```python
from build123d import *

# Parameters (mm, degrees)
F0_W      = 558.8
F0_H      = 330.2
F1_DEPTH  = 19.05
F2_W      = 38.1
F2_H      = 419.1
F2_H_2    = 203.2
F2_H_3    = 330.2
F3_DEPTH  = 88.9
F4_W      = 88.9
F4_H      = 88.9
F5_DEPTH  = 914.4
F6_W      = 38.1
F6_H      = 431.8
F6_W_2    = 431.8
F6_H_2    = 38.1
F7_DEPTH  = 139.7
F8_W      = 431.8
F8_H      = 69.85
F9_DEPTH  = 78.74
F10_W     = 431.8
F10_H     = 69.85
F11_DEPTH = 66.04
F12_W     = 431.8
F12_H     = 69.85
F13_DEPTH = 53.34
F14_W     = 431.8
F14_H     = 69.85
F15_DEPTH = 76.2


with BuildPart() as f1:
    # F0 (on Top) → F1 (new body)
    with BuildSketch(Plane.XY):
        Polygon((-907.6019599199, 71.2758600712), (-298.0019599199, -538.3241399288), (311.5980400801, -538.3241399288), (921.1980400801, 71.2758600712), (921.1980400801, 680.8758600712), (311.5980400801, 1290.4758600712), (-298.0019599199, 1290.4758600712), (-907.6019599199, 680.8758600712), align=None)
        with Locations((6.7980400801, 274.4758600712)):
            Rectangle(F0_W, F0_H, mode=Mode.SUBTRACT)
    extrude(amount=F1_DEPTH)

    # F2 (on face) → F3 (join)
    with BuildSketch(Plane(origin=(0, 0, 0), x_dir=(1, 0, 0), z_dir=(0, 0, -1))):
        with Locations((-278.9519599199, -890.4258600712)):
            Rectangle(F2_W, F2_H)
        with Locations((292.5480400801, -890.4258600712)):
            Rectangle(F2_W, F2_H)
        Polygon((-717.1019599199, -642.7758600712), (-717.1019599199, -680.8758600712), (-298.0019599199, -680.8758600712), (-259.9019599199, -680.8758600712), (273.4980400801, -680.8758600712), (311.5980400801, -680.8758600712), (730.6980400801, -680.8758600712), (730.6980400801, -642.7758600712), (273.4980400801, -642.7758600712), (235.3980400801, -642.7758600712), (-221.8019599199, -642.7758600712), (-259.9019599199, -642.7758600712), align=None)
        with Locations((-240.8519599199, -541.1758600712)):
            Rectangle(F2_W, F2_H_2)
        Polygon((-298.0019599199, -71.2758600712), (-717.1019599199, -71.2758600712), (-717.1019599199, -109.3758600712), (-272.6019599199, -109.3758600712), (-259.9019599199, -109.3758600712), (-221.8019599199, -109.3758600712), (235.3980400801, -109.3758600712), (273.4980400801, -109.3758600712), (286.1980400801, -109.3758600712), (730.6980400801, -109.3758600712), (730.6980400801, -71.2758600712), (311.5980400801, -71.2758600712), (273.4980400801, -71.2758600712), (-259.9019599199, -71.2758600712), align=None)
        with Locations((-278.9519599199, 138.2741399288)):
            Rectangle(F2_W, F2_H)
        with Locations((292.5480400801, 138.2741399288)):
            Rectangle(F2_W, F2_H)
        with Locations((254.4480400801, -541.1758600712)):
            Rectangle(F2_W, F2_H_2)
        with Locations((-240.8519599199, -274.4758600712)):
            Rectangle(F2_W, F2_H_3)
        with Locations((254.4480400801, -274.4758600712)):
            Rectangle(F2_W, F2_H_3)
    extrude(amount=F3_DEPTH)

    # F4 (on face) → F5 (join)
    with BuildSketch(Plane(origin=(0, 0, 0), x_dir=(1, 0, 0), z_dir=(0, 0, -1))):
        with Locations((775.1480400801, -636.4258600712)):
            Rectangle(F4_W, F4_H)
        with Locations((775.1480400801, -115.7258600712)):
            Rectangle(F4_W, F4_H)
        with Locations((267.1480400801, -1144.4258600712)):
            Rectangle(F4_W, F4_H)
        with Locations((-761.5519599199, -636.4258600712)):
            Rectangle(F4_W, F4_H)
        with Locations((-253.5519599199, -1144.4258600712)):
            Rectangle(F4_W, F4_H)
        with Locations((267.1480400801, 392.2741399288)):
            Rectangle(F4_W, F4_H)
        with Locations((-253.5519599199, 392.2741399288)):
            Rectangle(F4_W, F4_H)
        with Locations((-761.5519599199, -115.7258600712)):
            Rectangle(F4_W, F4_H)
    extrude(amount=F5_DEPTH)

    # F6 (on face) → F7 (join)
    with BuildSketch(Plane(origin=(0, 0, 0), x_dir=(1, 0, 0), z_dir=(0, 0, -1))):
        with Locations((800.5480400801, -376.0758600712)):
            Rectangle(F6_W, F6_H)
        with Locations((-786.9519599199, -376.0758600712)):
            Rectangle(F6_W, F6_H)
        with Locations((6.7980400801, -1169.8258600712)):
            Rectangle(F6_W_2, F6_H_2)
        with Locations((6.7980400801, 417.6741399288)):
            Rectangle(F6_W_2, F6_H_2)
    extrude(amount=F7_DEPTH)

    # F8 (on face) → F9 (cut)
    with BuildSketch(Plane.XZ.offset(436.7241399288)):
        with Locations((6.7980400801, -47.625)):
            Rectangle(F8_W, F8_H)
    extrude(amount=-F9_DEPTH, mode=Mode.SUBTRACT)

    # F10 (on face) → F11 (cut)
    with BuildSketch(Plane(origin=(-806.0019599199, 0, 0), x_dir=(0, -1, 0), z_dir=(-1, 0, 0))):
        with Locations((-376.0758600712, -47.625)):
            Rectangle(F10_W, F10_H)
    extrude(amount=-F11_DEPTH, mode=Mode.SUBTRACT)

    # F12 (on face) → F13 (cut)
    with BuildSketch(Plane.YZ.offset(819.5980400801)):
        with Locations((376.0758600712, -47.625)):
            Rectangle(F12_W, F12_H)
    extrude(amount=-F13_DEPTH, mode=Mode.SUBTRACT)

    # F14 (on face) → F15 (cut)
    with BuildSketch(Plane(origin=(0, 1188.8758600712, 0), x_dir=(-1, 0, 0), z_dir=(0, 1, 0))):
        with Locations((-6.7980400801, -47.625)):
            Rectangle(F14_W, F14_H)
    extrude(amount=-F15_DEPTH, mode=Mode.SUBTRACT)


solid = f1.part
```
Check sheet for the modelled part. Datum: model origin and axes. Units: mm. A direction names the side the tool comes from. Round coordinates to 2 decimals unless told otherwise and drop trailing zeros. Answer in a Markdown table with one row per item.
Q1. Release check for a two-part mould opening along Y. For faces 1 (the face through (-720, 71.276, -320)), 2 (the face through (-598.535, 989.943, 9.392)), 3 (the face through (-298.002, 1105, -320)), 4 (the face through (3, -160, 0)) record: released by +Y, released by -Y, zero draft, split by the parting line, or undercut.
Data:
| item | result |
|---|---|
| face 1 | released by -Y |
| face 2 | released by +Y |
| face 3 | zero draft |
| face 4 | undercut |
Q2. Set-up check for faces 5 (the face through (819.598, 603, -455)), 6 (the face through (-762, 636, -914.4)), 7 (the face through (311.598, 1105, -320)), 8 (the face through (-298.002, -351, -320)), 9 (the face through (-485, 642.776, -44)): record each of +Z, -Z, +X, -X, +Y, -Y from which the full face is reachable in a straight line by a thin tool's end or side.
Data:
| item | result |
|---|---|
| face 5 | -Z, +X, +Y, -Y |
| face 6 | -Z, +X, -X, +Y, -Y |
| face 7 | -Z, +X, +Y |
| face 8 | -Z, -X, -Y |
| face 9 | -Z |
Q3. Thickness scan on L1, parallel to Y at x = 816, z = -169.5; L2, parallel to X at y = 676.5, z = -626; L3, parallel to Y at x = -264.5, z = -798. Record the ranges inside material, lowest first.
Data:
| item | result |
|---|---|
| L1 | y = 71.28 to 160.18, 591.98 to 680.88 |
| L2 | x = -806 to -717.1, 730.7 to 819.6 |
| L3 | y = -436.72 to -347.82, 1099.98 to 1188.88 |
Q4. Go/stop test with flat-tipped pins: P1, Ø19, axis at x = -38, y = 1162.5, coming from the -Z side; P2, Ø1, axis at y = 134, z = -722, coming from the -X side; P3, Ø4, axis at x = 204.5, y = -149.5, coming from the -Z side. Record where each tip stops, or that it passes through.
Data:
| item | result |
|---|---|
| P1 | stops at z = -139.7 |
| P2 | stops at x = -806 |
| P3 | stops at z = 0 |
Q5. Sectioned sample at A-A on z = -766.5. Give the number of separate pieces and of enclosed holes in the cut face, then the cut area to 3 significant figures.
Data:
| item | result |
|---|---|
| separate pieces | 8 |
| enclosed holes | 0 |
| area | 63,200 mm^2 |
